For this review, take the finished solid that the model builds, in its own axes (mm). Face numbers are marked on the shaded views. A direction names the side the tool comes from. Coordinates: 2 decimals unless noted, no trailing zeros. Write each loop counter-clockwise with the first axis right and the second up, starting at its lowest first coordinate (ties: lowest second). Pieces come first, ordered by that corner, then holes.
1) We need section A-A on x = 5. Write out the cut boundary in (y, z) (3 decimals).
2) We need section C-C on z = 0.95. Write out the cut boundary in (x, y).
3) To check wall thickness, follow line 1 along Y through (x, z) = (0, 1.15); line 2 along Z through (x, y) = (3.5, -26) (3 decimals); line 3 along Y through (x, z) = (1.25, 0.15). State the ranges of each line that lie inside material, in increasing order.
4) We need section B-B on y = -6.5. Write out the cut boundary in (x, z).
5) For the marked faces 1 and 2, list the 3-axis set-ups (+Z, -Z, +X, -X, +Y, -Y) from which the entire face can be reached by the end or side of a thin tool; tool diameter is ignored.
Solid Edge part; units mm, degrees
sketch "Sketch1" plane through (0, 0, 0) normal (0, -1, 0) x (1, 0, 0)
  line L0 (0, 1.3) -> (5.8, 1.3)
  line L1 (5.8, -1.3) -> (0, -1.3)
  arc A0 (5.8, 1.3) -> (5.8, -1.3) centre (5.8, 0) cw
  arc A1 (0, -1.3) -> (0, 1.3) centre (0, 0) cw
extrude "Protrusion1" add sketch "Sketch1" along normal blind 25
sketch "Sketch2" plane through (2.6, -25, 0) normal (0, -1, 0) x (1, 0, 0)
  line L0 (-2.6, 0.325) -> (3.2, 0.325)
  line L1 (3.2, -0.325) -> (-2.6, -0.325)
  arc A0 (3.2, 0.325) -> (3.2, -0.325) centre (3.2, 0) cw
  arc A1 (-2.6, -0.325) -> (-2.6, 0.325) centre (-2.6, 0) cw
extrude "ExtrudedProtrusion_2" add sketch "Sketch2" along normal blind 2
fillet "Round_2" radius 0.2 4 edges at (2.9, -27, 0.325) (2.9, -27, -0.325) (6.125, -27, 0) (-0.325, -27, 0)
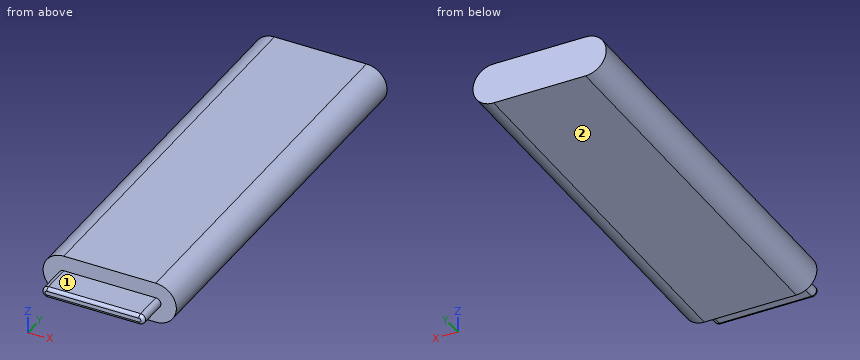
Result:
1. outline: (-27, -0.125) arc R0.2 ccw to (-26.8, -0.325) - (-25, -0.325) - (-25, -1.3) - (0, -1.3) - (0, 1.3) - (-25, 1.3) - (-25, 0.325) - (-26.8, 0.325) arc R0.2 ccw to (-27, 0.125) - close
2. outline: (-0.89, -25) - (6.69, -25) - (6.69, 0) - (-0.89, 0) - close
3. line 1: y = -25 to 0
3. line 2: z = -0.325 to 0.325
3. line 3: y = -27 to 0
4. outline: (0, -1.3) - (5.8, -1.3) arc R1.3 ccw to (5.8, 1.3) - (0, 1.3) arc R1.3 ccw to start
5. face 1: +Z, +X, -X, -Y
5. face 2: -Z, +X, -X, +Y, -Y
